The listing builds one solid part. Answer for the finished solid, in the listing's coordinates (mm). Face numbers are marked on the shaded views. A direction names the side the tool comes from. Give positions to 0.01 mm unless a question says otherwise; leave off trailing zeros. One line per question, with ' | ' between items.
from build123d import *

# Parameters (mm, degrees)
CROQUIS1_W              = 36.7
CROQUIS1_H              = 58
CROQUIS1_R              = 1.5
SALIENTE_EXTRUIR1_DEPTH = 1.3
CROQUIS2_W              = 35
CROQUIS2_H              = 40
SALIENTE_EXTRUIR2_DEPTH = 10.2
CORTAR_EXTRUIR1_DEPTH   = 54.572124281


with BuildPart() as part:
    # Croquis1 → Saliente-Extruir1 (new body)
    with BuildSketch(Plane(origin=(0, 0, 0), x_dir=(1, 0, 0), z_dir=(0, 1, 0))):
        Rectangle(CROQUIS1_W, CROQUIS1_H)
        with Locations(Location((15.35, 26, 0), (0, 0, 270))):
            Circle(CROQUIS1_R, mode=Mode.SUBTRACT)
        with Locations(Location((-15.35, 26, 0), (0, 0, 270))):
            Circle(CROQUIS1_R, mode=Mode.SUBTRACT)
        with Locations(Location((-15.35, -26, 0), (0, 0, 270))):
            Circle(CROQUIS1_R, mode=Mode.SUBTRACT)
        with Locations(Location((15.35, -26, 0), (0, 0, 270))):
            Circle(CROQUIS1_R, mode=Mode.SUBTRACT)
    extrude(amount=SALIENTE_EXTRUIR1_DEPTH)

    # Croquis2 → Saliente-Extruir2 (add)
    with BuildSketch(Plane(origin=(0, 1.3, 0), x_dir=(1, 0, 0), z_dir=(0, 1, 0))):
        Rectangle(CROQUIS2_W, CROQUIS2_H)
    extrude(amount=SALIENTE_EXTRUIR2_DEPTH)

    # Croquis3 → Cortar-Extruir1 (cut, through all)
    with BuildSketch(Plane.XY.offset(20)):
        with BuildLine():
            Line((-16.8, 11.1), (-15.914461251, 3.887865656))
            ThreePointArc((-15.914461251, 3.887865656), (-15.25, 3.3), (-14.585538749, 3.887865656))
            Line((-14.585538749, 3.887865656), (-13.7, 11.1))
            ThreePointArc((-13.7, 11.1), (-13.35, 11.45), (-13, 11.1))
            Line((-13, 11.1), (-12.114461251, 3.887865656))
            ThreePointArc((-12.114461251, 3.887865656), (-11.45, 3.3), (-10.785538749, 3.887865656))
            Line((-10.785538749, 3.887865656), (-9.9, 11.1))
            ThreePointArc((-9.9, 11.1), (-9.55, 11.45), (-9.2, 11.1))
            Line((-9.2, 11.1), (-8.314461251, 3.887865656))
            ThreePointArc((-8.314461251, 3.887865656), (-7.65, 3.3), (-6.985538749, 3.887865656))
            Line((-6.985538749, 3.887865656), (-6.1, 11.1))
            ThreePointArc((-6.1, 11.1), (-5.75, 11.45), (-5.4, 11.1))
            Line((-5.4, 11.1), (-4.514461251, 3.887865656))
            ThreePointArc((-4.514461251, 3.887865656), (-3.85, 3.3), (-3.185538749, 3.887865656))
            Line((-3.185538749, 3.887865656), (-2.3, 11.1))
            ThreePointArc((-2.3, 11.1), (-1.95, 11.45), (-1.6, 11.1))
            Line((-1.6, 11.1), (-0.714461251, 3.887865656))
            ThreePointArc((-0.714461251, 3.887865656), (-0.05, 3.3), (0.614461251, 3.887865656))
            Line((0.614461251, 3.887865656), (1.5, 11.1))
            ThreePointArc((1.5, 11.1), (1.85, 11.45), (2.2, 11.1))
            Line((2.2, 11.1), (3.085538749, 3.887865656))
            ThreePointArc((3.085538749, 3.887865656), (3.75, 3.3), (4.414461251, 3.887865656))
            Line((4.414461251, 3.887865656), (5.3, 11.1))
            ThreePointArc((5.3, 11.1), (5.65, 11.45), (6, 11.1))
            Line((6, 11.1), (6.885538749, 3.887865656))
            ThreePointArc((6.885538749, 3.887865656), (7.55, 3.3), (8.214461251, 3.887865656))
            Line((8.214461251, 3.887865656), (9.1, 11.1))
            ThreePointArc((9.1, 11.1), (9.45, 11.45), (9.8, 11.1))
            Line((9.8, 11.1), (10.685538749, 3.887865656))
            ThreePointArc((10.685538749, 3.887865656), (11.35, 3.3), (12.014461251, 3.887865656))
            Line((12.014461251, 3.887865656), (12.9, 11.1))
            ThreePointArc((12.9, 11.1), (13.25, 11.45), (13.6, 11.1))
            Line((13.6, 11.1), (14.485538749, 3.887865656))
            ThreePointArc((14.485538749, 3.887865656), (15.15, 3.3), (15.814461251, 3.887865656))
            Line((15.814461251, 3.887865656), (16.7, 11.1))
            ThreePointArc((16.7, 11.1), (17.123486281, 11.450780489), (17.5, 11.05))
            Line((17.5, 11.05), (17.5, 11.5))
            Line((17.5, 11.5), (-17.5, 11.5))
            Line((-17.5, 11.5), (-17.5, 11.1))
            ThreePointArc((-17.5, 11.1), (-17.15, 11.45), (-16.8, 11.1))
        make_face()
    extrude(amount=-CORTAR_EXTRUIR1_DEPTH, mode=Mode.SUBTRACT)


solid = part.part
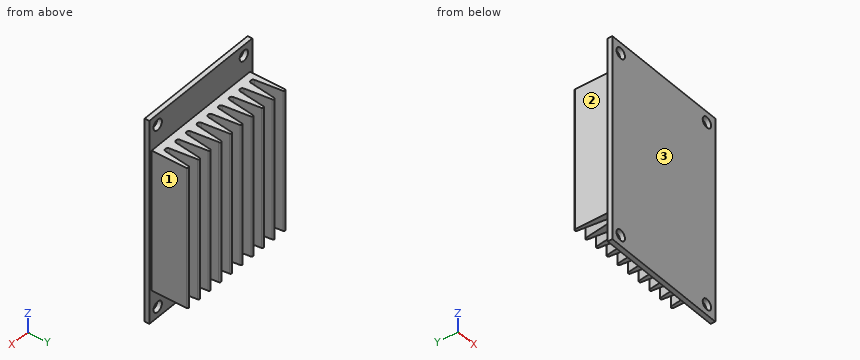
Item 1: A tool of negligible diameter and unlimited length cuts with its end or side. For the marked faces 1, 2 and 3, from which of +Z, -Z, +X, -X, +Y, -Y can it reach the whole face along a straight path? Write none if from no direction.
Answers below:
face 1: +Z, -Z, +X, +Y | face 2: +Z, -Z, -X, +Y | face 3: +Z, -Z, +X, -X, -Y
Item 2: Find section A-A (y = 5). Count the separate pieces of the cut face and the enclosed holes in it, then the cut area to 3 significant figures.
Answers below:
separate pieces: 10 | enclosed holes: 0 | area: 823 mm²
Item 3: Flat-ended cylindrical pins translate along their axes: pin 1 (5 mm diameter, centred on y = 5, z = 20, fed in from +X); pin 2 (4 mm diameter, centred on x = 5.5, y = 3.5, fed in from -Z); pin 3 (3 mm diameter, centred on y = 5.5, z = 18, fed in from -X); pin 4 (1.8 mm diameter, centred on x = 15.35, z = 26, fed in from -Y). Find the tip coordinate at first contact, or state that the pin passes through.
Answers below:
pin 1: x = 17.5 | pin 2: z = -20 | pin 3: x = -17.5 | pin 4: through
Item 4: Consider line 1 (X direction, y = 0.3, z = 26); line 2 (Z direction, x = -10, y = 9); line 3 (X direction, y = 2.25, z = 19.5). Determine where each line is inside the solid, lowest interval first. Write a range as [from, to].
Answers below:
line 1: [-18.35, -16.85], [-13.85, 13.85], [16.85, 18.35] | line 2: [-20, 20] | line 3: [-17.5, 17.5]
